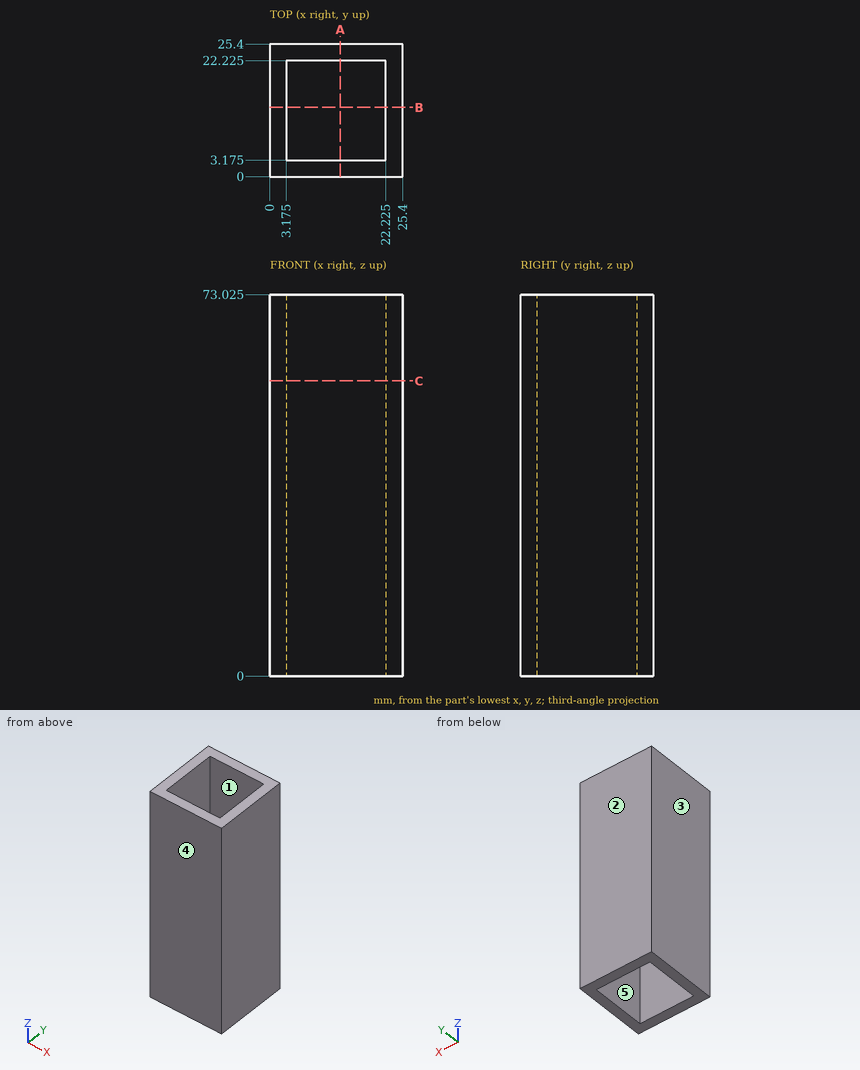
Geometry check sheet. Reference: drawing and pictorial views, mm from the part's lowest x, y, z. A direction names the side the tool comes from. Give positions to 0.01 mm unless a question says otherwise; leave off trailing zeros. Loops run counter-clockwise (first coordinate to the right, second up) from the corner with the lowest first, then second, coordinate; pieces in that order, holes last. Notation, with made-up numbers: M 21,62.5 L 56,62.5 A33 cw 56,92.5 Z; hole C 43.5,74 d7. An arc over 180 degrees is marked long. Use a Markdown table: item, result. Add a question column.
Q1. Scan line: line 1 along Y through (x, z) = (16.5, 44) (3 decimals). Record every from-to range of solid material in increasing order. Write a range as [from, to].
Q2. Mould release check, pull along Y, two halves, no side actions. Record for the marked faces 1, 2 and 3: pulls with the +Y half, pulls with the -Y half, needs draft (parallel to the pull), parting line crosses it, or undercut.
Q3. Tool access check on the marked faces 4 and 5. Record the directions out of +Z, -Z, +X, -X, +Y, -Y that give a thin tool (end or side, any length) a straight path to the whole face; none if there is none.
Q4. Sectioned sample at A-A, the plane x = 13.5. Record the cut outline in (y, z) (3 decimals), then the cut area to 3 significant figures.
Q5. Sectioned sample at C-C, the plane z = 56.5. Record the cut outline in (x, y) (3 decimals).
Verdict:
| question | item | result |
|---|---|---|
| 1 | line 1 | [0, 3.175], [22.225, 25.4] |
| 2 | face 1 | undercut |
| 2 | face 2 | pulls with the +Y half |
| 2 | face 3 | needs draft |
| 3 | face 4 | +Z, -Z, +X, -X, -Y |
| 3 | face 5 | +Z, -Z |
| 4 | outline | M 0,0 L 3.175,0 L 3.175,73.025 L 0,73.025 Z; M 22.225,0 L 25.4,0 L 25.4,73.025 L 22.225,73.025 Z |
| 4 | area | 464 mm^2 |
| 5 | outline | M 0,0 L 25.4,0 L 25.4,25.4 L 0,25.4 Z; hole M 3.175,3.175 L 22.225,3.175 L 22.225,22.225 L 3.175,22.225 Z |
